Geometry: final body of the model. Coordinates: model frame, mm. A direction names the side the tool comes from. Round coordinates to 2 decimals unless told otherwise and drop trailing zeros. Write each loop counter-clockwise with the first axis right and the second up, starting at its lowest first coordinate (ties: lowest second). Pieces come first, ordered by that corner, then holes. Notation, with made-up numbers: M 85.5,78 L 123.5,78 A33 ccw 123.5,109 Z; hole C -13.5,-25 d3. An arc over 180 degrees is marked long. Use one line per item in the form item = value. Start each with the question number.
Item 1: Pin query (flat end, axial travel): pin 1 Ø2 at (x, z) = (6.5, 1) entering from -Y; pin 2 Ø1 at (y, z) = (8, 5.5) entering from -X; pin 3 Ø4 at (x, y) = (-5.5, 5.5) entering from +Z. Return the tip coordinate at first contact, or that it passes through.
Item 2: Section query A-A (x = 0). Return loops of the section in (y, z).
Item 3: Section query D-D (y = 8.25). Return loops of the section in (x, z), and give its area (3 significant figures).
Item 4: Section query C-C (z = 3). Return loops of the section in (x, y).
Item 5: Pull-direction query (Y, two-part tool) for faces 4 (the cylindrical face through (-2.38, 10.74, 3.45)), 5 (the cylindrical face through (-0.867, 3.905, 3.451)), 6 (the flat face through (2, -10, 7)); classes: pulls with the +Y half, pulls with the -Y half, needs draft (parallel to the pull), parting line crosses it, or undercut.
Item 6: Reachability of faces 1 (the flat face through (2, -10, 0)), 2 (the cylindrical face through (-2.17, -9.76, 6.51)), 3 (the cylindrical face through (1.08, -4.88, 0.49)) from +Z, -Z, +X, -X, +Y, -Y: full face, straight path, thin tool, end or side. Return the list, or none.
Item 7: Ray query, probe 1 along Y at (x, z) = (0, 6.3); probe 2 along Y at (x, z) = (0, 3.75); probe 3 along Z at (x, y) = (5.5, -6). Return the intervals inside material, ascending.
Autodesk Inventor part; units mm, degrees
ref_plane "YZ Plane" through (0, 0, 0) normal (1, 0, 0) x (0, 1, 0)
ref_plane "XZ Plane" through (0, 0, 0) normal (0, 1, 0) x (-1, 0, 0)
ref_plane "XY Plane" through (0, 0, 0) normal (0, 0, 1) x (1, 0, 0)
sketch "Эскиз1" plane through (0, 0, 0) normal (0, 0, 1) x (1, 0, 0)
  circle A0 centre (0, 0) radius 4
  circle A1 centre (0, 0) radius 11
  dimension "d0" = 8
  dimension "d1" = 22
extrude "Выдавливание1" add sketch "Эскиз1" along normal blind 7
sketch "Эскиз3" plane through (0, 0, 7) normal (0, 0, 1) x (1, 0, 0)
  circle A0 centre (0, 0) radius 4
  circle A1 centre (0, 0) radius 4
  circle A2 centre (0, 0) radius 5
  circle A3 centre (0, 0) radius 10
  circle A4 centre (0, 0) radius 11
  dimension "d8" = 10
  dimension "d9" = 20
  dimension "d10" = 22
  dimension "d11" = 8
extrude "Выдавливание3" cut sketch "Эскиз3" against normal blind 1 contours A3
sketch "Эскиз4" plane through (0, 0, 0) normal (0, 0, -1) x (-1, 0, 0)
  circle A0 centre (0, 0) radius 4
  circle A1 centre (0, 0) radius 5
  circle A2 centre (0, 0) radius 11
  circle A3 centre (0, 0) radius 10
  dimension "d14" = 20
  dimension "d15" = 8
  dimension "d16" = 10
  dimension "d17" = 22
extrude "Выдавливание4" cut sketch "Эскиз4" against normal blind 1 contours A3
properties part number "Подшипник"
Working result:
q1.pin_1 = -9.53
q1.pin_2 = -8.05
q1.pin_3 = 6
q2.outline = M -11,0 L -10,0 L -10,1 L -5,1 L -5,0 L -4,0 L -4,7 L -5,7 L -5,6 L -10,6 L -10,7 L -11,7 Z; M 4,0 L 5,0 L 5,1 L 10,1 L 10,0 L 11,0 L 11,7 L 10,7 L 10,6 L 5,6 L 5,7 L 4,7 Z
q3.outline = M -7.28,0 L -5.65,0 L -5.65,1 L 5.65,1 L 5.65,0 L 7.28,0 L 7.28,7 L 5.65,7 L 5.65,6 L -5.65,6 L -5.65,7 L -7.28,7 Z
q3.area = 79.3 mm²
q4.outline = C 0,0 d22; hole C 0,0 d8
q5.face_4 = parting line crosses it
q5.face_5 = undercut
q5.face_6 = needs draft
q6.face_1 = -Z, +X, -X, +Y, -Y
q6.face_2 = +Z
q6.face_3 = -Z
q7.probe_1 = -11 to -10, -5 to -4, 4 to 5, 10 to 11
q7.probe_2 = -11 to -4, 4 to 11
q7.probe_3 = 1 to 6
